Here's how the part is built. I have some questions about the finished solid (model axes, mm). Round coordinates to 2 decimals unless told otherwise and drop trailing zeros. Loops run counter-clockwise (first coordinate to the right, second up) from the corner with the lowest first, then second, coordinate; pieces in that order, holes last. Notation, with made-up numbers: M -4,-29 L 55,-29 A18 ccw 55,-23 Z; hole C 79,64 d8. An arc over 180 degrees is marked long. Write item = value, one per line. Start each with the question number.
Autodesk Inventor part; units mm, degrees
ref_plane "Work Plane2" through (-53.25, -178, -67.8971) normal (0, -1, 0) x (0.8660254, 0, -0.5)
ref_plane "Work Plane5" through (-46.3218, -178, -67.8971) normal (0, -1, 0) x (0.8660254, 0, -0.5)
ref_plane "YZ Plane" through (0, 0, 0) normal (1, 0, 0) x (0, 1, 0)
ref_plane "Work Plane1" through (14.6553, 0, -25.7817) normal (0, 1, 0) x (-0.8660254, 0, 0.5)
ref_plane "Work Plane2" through (-53.25, -178, -67.8971) normal (0, -1, 0) x (0.8660254, 0, -0.5)
ref_plane "Work Plane3" through (14.6553, 0, -25.7817) normal (0, 1, 0) x (-0.8660254, 0, 0.5)
ref_plane "Work Plane4" through (-55.7811, 0, -1.2811) normal (0, 1, 0) x (0.5, 0, 0.8660254)
sketch "Sketch4" plane through (-55.7811, 0, -1.2811) normal (0, 1, 0) x (0.5, 0, 0.8660254)
  line L0 (3.5, 3.5) -> (-1, 3.5)
  line L1 (-1, 3.5) -> (-1, -0.5)
  line L2 (-1, -0.5) -> (-4.5, -0.5)
  line L3 (-4.5, -0.5) -> (-4.5, -14.5)
  line L4 (-4.5, -14.5) -> (4.5, -0.5)
  line L5 (4.5, -0.5) -> (3.5, -0.5)
  line L6 (3.5, -0.5) -> (3.5, 3.5)
  line L7 (8.1188, 11.5) -> (29, 47.6673)
  line L8 (29, 47.6673) -> (3.5, 3.5)
  line L9 (3.5, 1.7679) -> (30, 47.6673)
  line L10 (30, 47.6673) -> (29, 47.6673)
  point P0 (29, 47.6673)
  dimension "d10" = 1
ref_plane "Work Plane5" through (-46.3218, -178, -67.8971) normal (0, -1, 0) x (0.8660254, 0, -0.5)
extrude "Extrusion2" add sketch "Sketch4" against normal up to surface (178 mm away) contours L8 L7 L10 L9 L6
sketch "Sketch5" plane through (-52.5, 0, 0.866) normal (0, 0, 1) x (1, 0, 0)
  circle A0 centre (42.0594, -3) radius 2.3
  circle A1 centre (21.1782, -3) radius 2.3
  circle A2 centre (30.6045, -58.5) radius 2.3
  circle A3 centre (45.2015, -58.5) radius 2.3
  circle A4 centre (30.6045, -119.5) radius 2.3
  circle A5 centre (45.2015, -119.5) radius 2.3
  circle A6 centre (21.1782, -175) radius 2.3
  circle A7 centre (42.0594, -175) radius 2.3
  point P0 (52.5, 0)
hole "Hole2" at (-10.4406, -3, 0.866) at (-31.3218, -3, 0.866) at (-7.2985, -58.5, 0.866) at (-21.8955, -58.5, 0.866) at (-7.2985, -119.5, 0.866) at (-21.8955, -119.5, 0.866) at (-31.3218, -175, 0.866) at (-10.4406, -175, 0.866) direction (0, 0, -1) diameter 3.6 end through all countersink diameter 6.7 countersink angle 90
properties part number "frobt" material "Nylon 6/6"
Item 1: I want a section at A-A, the plane y = -119.5. List the corners of the cut face in (x, z) for me, then the cut area to 3 significant figures.
Item 2: Please list where these lines run through material, in increasing order: line 1 (Y direction, x = -23, z = 0.8); line 2 (Y direction, x = -9, z = 0.55); line 3 (Y direction, x = -7.5, z = 0.25). Write a range as [from, to].
Item 3: I want a section at B-B, the plane y = -49.5. List the corners of the cut face in (x, z) for me, then the cut area to 3 significant figures.
Item 4: We'd pull the mould along X, two halves only. Please class faces 1 (the conical face through (-10.32, -172.37, 0.15)), 2 (the flat face through (-26, -88, 0.866)): released by +X, released by -X, zero draft, split by the parting line, or undercut.
Worked out:
q1.outline = M -52.5,0.87 L -51,0 L -24.38,0 L -25.25,0.87 Z; M -19.41,0 L -9.78,0 L -10.65,0.87 L -18.55,0.87 Z; M -4.81,0 L 0,0 L 0.5,0.87 L -3.95,0.87 Z
q1.area = 34.9 mm2
q2.line_1 = [-178, -122.59], [-116.41, -61.59], [-55.41, 0]
q2.line_2 = [-178, -177.67], [-172.33, -122.01], [-116.99, -61.01], [-55.99, -5.67], [-0.33, 0]
q2.line_3 = [-178, -122.23], [-116.77, -61.23], [-55.77, 0]
q3.outline = M -52.5,0.87 L -51,0 L 0,0 L 0.5,0.87 Z
q3.area = 45.0 mm2
q4.face_1 = undercut
q4.face_2 = zero draft
